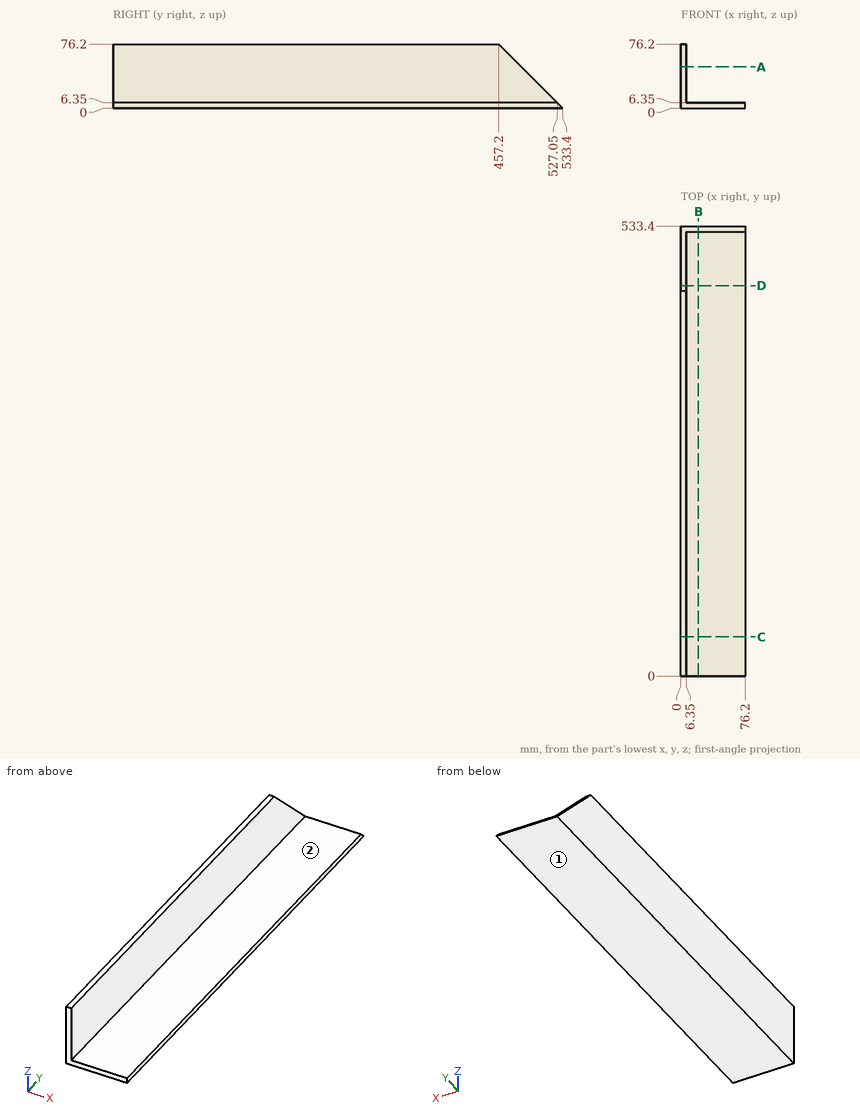
For this review, use the dimensioned drawing (mm, ordinates from the lowest corner) and the shaded views. A direction names the side the tool comes from. Round coordinates to 2 decimals unless told otherwise and drop trailing zeros. Order: outer loops, then holes, each group sorted by start corner. A loop starts at its lowest first (then second) coordinate and runs counter-clockwise, first axis right, second up.
1) Clearance check with flat-ended pins moving along their axes: pin 1 Ø1.5 at (x, y) = (68.5, 256.5) entering from -Z; pin 2 Ø6 at (y, z) = (290.5, 27) entering from +X; pin 3 Ø3 at (x, y) = (64, 473.5) entering from +Z. State where each tip first meets the part, or that it passes through.
The answers:
pin 1: stops at z = 0
pin 2: stops at x = 6.35
pin 3: stops at z = 6.35
2) Consider section C-C (y = 46.5). State the section outline as (x, z) points, plus the area to 3 significant figures.
The answers:
outline: (0, 0) - (76.2, 0) - (76.2, 6.35) - (6.35, 6.35) - (6.35, 76.2) - (0, 76.2) - close
area: 927 mm2
3) Consider section A-A (z = 49). State the section outline as (x, y) points.
The answers:
outline: (0, 0) - (6.35, 0) - (6.35, 484.4) - (0, 484.4) - close
4) Consider section B-B (x = 21). State the section outline as (y, z) points.
The answers:
outline: (0, 0) - (533.4, 0) - (527.05, 6.35) - (0, 6.35) - close
5) Machinability: for the marked faces 1 and 2, which of the approach directions +Z, -Z, +X, -X, +Y, -Y give a long, thin tool a straight path to every point of the face, cutting with its end or side? Answer none if there is none.
The answers:
face 1: -Z, +X, -X, +Y, -Y
face 2: +Z, +X, +Y, -Y
6) Consider section D-D (y = 463). State the section outline as (x, z) points.
The answers:
outline: (0, 0) - (76.2, 0) - (76.2, 6.35) - (6.35, 6.35) - (6.35, 70.4) - (0, 70.4) - close
7) For L1, parallel to Z at x = 20, y = 282; L2, parallel to Y at x = 10.5, z = 6, list the stretches that pass through material, from the lowest coordinate up.
The answers:
L1: z = 0 to 6.35
L2: y = 0 to 527.4
